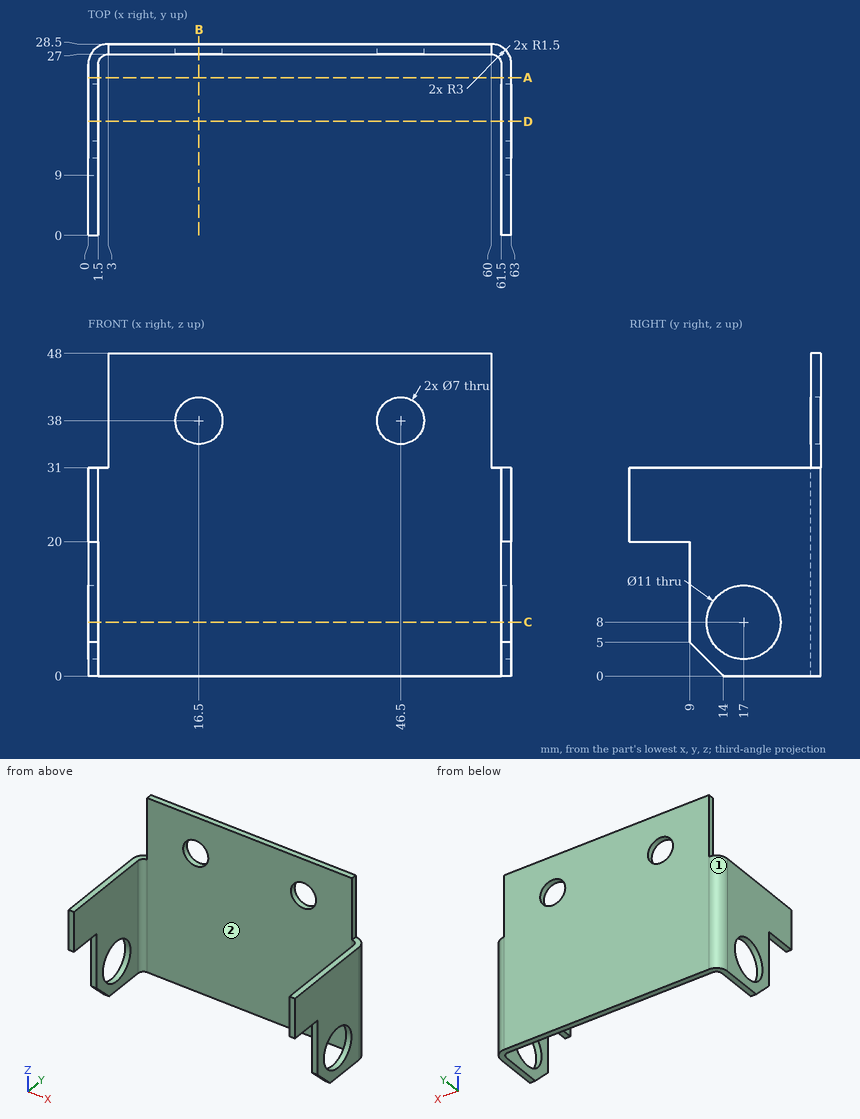
Geometry: see drawing. Coordinates: mm, zero at the bounding-box minimum. A direction names the side the tool comes from. Coordinates: 2 decimals unless noted, no trailing zeros. Order: outer loops, then holes, each group sorted by start corner. A loop starts at its lowest first (then second) coordinate and runs counter-clockwise, first axis right, second up. Notation, with made-up numbers: M 2,79 L 53,79 A22 ccw 53,110 Z; hole C 62.25,89 d4. An arc over 180 degrees is marked long. Answer in a Markdown table with one row per item. Add a question column.
Q1. Reachability of the marked faces 1 and 2 from +Z, -Z, +X, -X, +Y, -Y: full face, straight path, thin tool, end or side. Return the list, or none.
Q2. Contact query for flat-ended pins moving along their axis: P1, Ø0.8, axis at x = 1, y = 6, coming from the -Z side; P2, Ø9, axis at y = 17, z = 8, coming from the +X side; P3, Ø0.8, axis at x = 1, z = 9.5, coming from the -Y side; P4, Ø3.5, axis at x = 1.5, y = 9, coming from the +Z side. Output: stop coordinate, or through.
Q3. Section query D-D on y = 17. Return the cut outline in (x, z), and give its area (3 significant figures).
Q4. Section query A-A on y = 23.5. Return the cut outline in (x, z).
Q5. Section query B-B on x = 16.5. Return the cut outline in (y, z).
Q6. Section query C-C on z = 8. Return the cut outline in (x, y).
Q7. Line query: L1, parallel to X at y = 27.5, z = 38; L2, parallel to X at y = 21, z = 26; L3, parallel to Z at x = 46.5, y = 27.55. Output: solid intervals per line, ascending.
Completed:
| question | item | result |
|---|---|---|
| 1 | face 1 | +Z, -Z, -X, +Y |
| 1 | face 2 | +Z, -Z, -Y |
| 2 | P1 | stops at z = 20 |
| 2 | P2 | passes through |
| 2 | P3 | stops at y = 9 |
| 2 | P4 | stops at z = 31 |
| 3 | outline | M 0,0 L 1.5,0 L 1.5,2.5 L 0,2.5 Z; M 0,13.5 L 1.5,13.5 L 1.5,31 L 0,31 Z; M 61.5,0 L 63,0 L 63,2.5 L 61.5,2.5 Z; M 61.5,13.5 L 63,13.5 L 63,31 L 61.5,31 Z |
| 3 | area | 60.0 mm2 |
| 4 | outline | M 0,0 L 1.5,0 L 1.5,31 L 0,31 Z; M 61.5,0 L 63,0 L 63,31 L 61.5,31 Z |
| 5 | outline | M 27,0 L 28.5,0 L 28.5,34.5 L 27,34.5 Z; M 27,41.5 L 28.5,41.5 L 28.5,48 L 27,48 Z |
| 6 | outline | M 0,9 L 1.5,9 L 1.5,11.5 L 0,11.5 Z; M 0,22.5 L 1.5,22.5 L 1.5,25.5 A1.5 cw 3,27 L 60,27 A1.5 cw 61.5,25.5 L 61.5,22.5 L 63,22.5 L 63,25.5 A3 ccw 60,28.5 L 3,28.5 A3 ccw 0,25.5 Z; M 61.5,9 L 63,9 L 63,11.5 L 61.5,11.5 Z |
| 7 | L1 | x = 3 to 13, 20 to 43, 50 to 60 |
| 7 | L2 | x = 0 to 1.5, 61.5 to 63 |
| 7 | L3 | z = 0 to 34.5, 41.5 to 48 |
